Here's how the part is built. I have some questions about the finished solid (model axes, mm). Give positions to 0.01 mm unless a question says otherwise; leave off trailing zeros. Loops run counter-clockwise (first coordinate to the right, second up) from the corner with the lowest first, then second, coordinate; pieces in that order, holes last. Notation, with made-up numbers: M 48,33.25 L 54,33.25 A28 ccw 54,53.25 Z; hole C -27,16 d3. An arc over 180 degrees is marked long. Answer as CSV lines item,"result". Start each with the question number.
Item 1: If I drill on line 1 along Y through (x, z) = (0, -0.9); line 2 along Y through (x, z) = (1, -1.45); line 3 along X through (y, z) = (1, -0.3), over which ranges is the centre line in solid material (lowest first)? Write a range as from..to.
Item 2: I want a section at A-A on z = -1.2. List the corners of the cut face in (x, y) for me, plus the area to 3 significant figures.
Item 3: I want a section at C-C on z = -2.45. List the corners of the cut face in (x, y) for me, plus the area to 3 significant figures.
Item 4: I want a section at B-B on x = 0. List the corners of the cut face in (y, z) for me, plus the area to 3 significant figures.
Item 5: Will these pins go through, and if not, where does the flat tip stop? P1, Ø3, axis at x = 2, y = 1, coming from the -Z side; P2, Ø1.5, axis at y = 2, z = -1, coming from the +X side; P3, Ø1, axis at y = 2, z = -1.5, coming from the -X side.
from build123d import *

# Parameters (mm, degrees)
BASENUTSKE_R            = 2.5
BASENUT_DEPTH           = 2.7
SKETCH6_OUTSIDE_W       = 40.346
SKETCH6_OUTSIDE_H       = 39.108
SKETCH6_OUTSIDE_R       = 3.8
CUT_EXTRUDE2_DEPTH      = 7.68006986
CUT_EXTRUDE2_DRAFT      = -60
MIRROR1_COPY_1_SKETCH_W = 40.346
MIRROR1_COPY_1_SKETCH_H = 39.108
MIRROR1_COPY_1_SKETCH_R = 3.8
MIRROR1_COPY_1_DEPTH    = 7.68006986
MIRROR1_COPY_1_DRAFT    = -60


with BuildPart() as part:
    # BaseNutSke → BaseNut (new body)
    with BuildSketch(Plane.XY):
        Polygon((2.309401077, -4), (-2.309401077, -4), (-4.618802154, 0), (-2.309401077, 4), (2.309401077, 4), (4.618802154, 0), align=None)
        Circle(BASENUTSKE_R, mode=Mode.SUBTRACT)
    extrude(amount=-BASENUT_DEPTH)


with BuildPart() as cut_extrude2_tool:
    # Sketch6 outside → Cut-Extrude2 (with draft: the straight prism first)
    with BuildSketch(Plane(origin=(0, 0, -2.7), x_dir=(-1, 0, 0), z_dir=(0, 0, -1))):
        Rectangle(SKETCH6_OUTSIDE_W, SKETCH6_OUTSIDE_H)
        Circle(SKETCH6_OUTSIDE_R, mode=Mode.SUBTRACT)
    extrude(amount=-CUT_EXTRUDE2_DEPTH)
    # Cut-Extrude2: the draft: its side faces are tilted about the plane it starts from
    cut_extrude2_sides = [cut_extrude2_tool.faces().sort_by_distance(p)[0] for p in [
        (0, -19.554, 1.14003493),
        (-20.173, 0, 1.14003493),
        (0, 19.554, 1.14003493),
        (20.173, 0, 1.14003493),
        (3.8, 0, 1.14003493),
    ]]
    draft(cut_extrude2_sides, Plane(origin=(0, 0, -2.7), x_dir=(-1, 0, 0), z_dir=(0, 0, -1)), CUT_EXTRUDE2_DRAFT)


with BuildPart() as part_1:
    add(part.part)

    # Cut-Extrude2: cut by cut_extrude2_tool
    add(cut_extrude2_tool.part, mode=Mode.SUBTRACT)


with BuildPart() as mirror1_copy_1_tool:
    # Mirror1 copy 1 sketch → Mirror1 copy 1 (with draft: the straight prism first)
    with BuildSketch(Plane(origin=(0, 0, 0), x_dir=(-1, 0, 0), z_dir=(0, 0, 1))):
        Rectangle(MIRROR1_COPY_1_SKETCH_W, MIRROR1_COPY_1_SKETCH_H)
        Circle(MIRROR1_COPY_1_SKETCH_R, mode=Mode.SUBTRACT)
    extrude(amount=-MIRROR1_COPY_1_DEPTH)
    # Mirror1 copy 1: the draft: its side faces are tilted about the plane it starts from
    mirror1_copy_1_sides = [mirror1_copy_1_tool.faces().sort_by_distance(p)[0] for p in [
        (0, -19.554, -3.84003493),
        (-20.173, 0, -3.84003493),
        (0, 19.554, -3.84003493),
        (20.173, 0, -3.84003493),
        (3.8, 0, -3.84003493),
    ]]
    draft(mirror1_copy_1_sides, Plane(origin=(0, 0, 0), x_dir=(-1, 0, 0), z_dir=(0, 0, 1)), MIRROR1_COPY_1_DRAFT)


with BuildPart() as part_2:
    add(part_1.part)

    # Mirror1 copy 1: cut by mirror1_copy_1_tool
    add(mirror1_copy_1_tool.part, mode=Mode.SUBTRACT)


solid = part_2.part
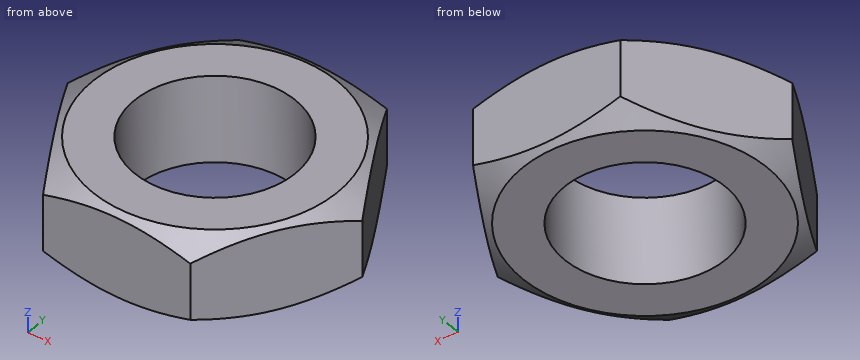
Result:
1,line 1,"-4..-2.5, 2.5..4"
1,line 2,"-4..-2.29, 2.29..4"
1,line 3,"-4.04..-2.29, 2.29..4.04"
2,outline,"M -4.62,0 L -2.31,-4 L 2.31,-4 L 4.62,0 L 2.31,4 L -2.31,4 Z; hole C 0,0 d5"
2,area,"35.8 mm^2"
3,outline,"M -4.16,-0.8 L -2.77,-3.2 A4.23 ccw -1.39,-4 L 1.39,-4 A4.23 ccw 2.77,-3.2 L 4.16,-0.8 A4.23 ccw 4.16,0.8 L 2.77,3.2 A4.23 ccw 1.39,4 L -1.39,4 A4.23 ccw -2.77,3.2 L -4.16,0.8 A4.23 ccw Z; hole C 0,0 d5"
3,area,"34.1 mm^2"
4,outline,"M -4,-2.58 L -3.8,-2.7 L -2.5,-2.7 L -2.5,0 L -3.8,0 L -4,-0.12 Z; M 2.5,-2.7 L 3.8,-2.7 L 4,-2.58 L 4,-0.12 L 3.8,0 L 2.5,0 Z"
4,area,"8.05 mm^2"
5,P1,"z = -2.7"
5,P2,"x = 3.9"
5,P3,"x = -3.75"
